CAD build for the part. Positions are in the model's coordinates, mm. A direction names the side the tool comes from. Round coordinates to 2 decimals unless told otherwise and drop trailing zeros. Write each loop counter-clockwise with the first axis right and the second up, starting at its lowest first coordinate (ties: lowest second). Pieces come first, ordered by that corner, then holes. Notation, with made-up numbers: (76, 74) -> (119, 74) arc R28 ccw to (119, 104) -> close; hole circle Ø8 at (5.5, 12). An arc over 180 degrees is marked (long way). Put each result on its own line as item: value. Start each with the question number.
1. Flat gauge pins, fed straight in: P1, Ø0.9, axis at y = 3.175, z = -50.8, coming from the +X side; P2, Ø0.8, axis at y = 3, z = -51, coming from the -X side; P3, Ø2, axis at x = 9.5, z = -13, coming from the -Y side. Where does each tip first touch, or does it go through?
2. Saw through at B-B on z = 0. List the corners of the cut face in (x, y).
3. Saw through at A-A on x = 0. List the corners of the cut face in (y, z).
4. Saw through at C-C on x = -15. List the corners of the cut face in (y, z), and give its area (3 significant figures).
5. Drill centre lines: line 1 (Z direction, x = 0, y = 5); line 2 (Y direction, x = 0, z = -70.75); line 3 (Z direction, x = 0, y = 4). Where is each one in solid material? Low to high. Write a range as from..to.
6. 3-axis set-ups, long thin cutter, end or side, ignore diameter. For faces 4 (the flat face through (-14, 6.35, -18)), 5 (the cylindrical face through (-0.93, 4.63, -73.07)): which of +Z, -Z, +X, -X, +Y, -Y reach the whole face in a straight line?
7. Pull direction Y, two halves, no side cores. Call faces 1 (the flat face through (58.75, 3, 1)), 2 (the flat face through (-14, 0, -18)), 3 (the flat face through (0, 3, -69.85)): pulls with the +Y half, pulls with the -Y half, needs draft (parallel to the pull), parting line crosses it, or undercut.
from build123d import *

# Parameters (mm, degrees)
SKETCH1_W           = 117.5004
SKETCH1_H           = 152.4
SKETCH1_R           = 19.05
BOSS_EXTRUDE1_DEPTH = 6.35
SKETCH3_R           = 0.7874
CUT_EXTRUDE1_DEPTH  = 0.508
SKETCH4_R           = 0.7874
CUT_EXTRUDE2_DEPTH  = 0.508
SKETCH5_R           = 1.7272
CUT_EXTRUDE3_DEPTH  = 6.35


with BuildPart() as part:
    # Sketch1 → Boss-Extrude1 (new body)
    with BuildSketch(Plane(origin=(0, 0, 0), x_dir=(1, 0, 0), z_dir=(0, 1, 0))):
        Rectangle(SKETCH1_W, SKETCH1_H)
        Circle(SKETCH1_R, mode=Mode.SUBTRACT)
    extrude(amount=BOSS_EXTRUDE1_DEPTH)

    # Sketch3 → Cut-Extrude1 (cut)
    with BuildSketch(Plane.ZY.offset(58.7502)):
        with Locations((-50.8, 3.175)):
            Circle(SKETCH3_R)
    extrude(amount=-CUT_EXTRUDE1_DEPTH, mode=Mode.SUBTRACT)

    # Sketch4 → Cut-Extrude2 (cut)
    with BuildSketch(Plane(origin=(58.7502, 0, 0), x_dir=(0, 0, -1), z_dir=(1, 0, 0))):
        with Locations((50.8, 3.175)):
            Circle(SKETCH4_R)
    extrude(amount=-CUT_EXTRUDE2_DEPTH, mode=Mode.SUBTRACT)

    # Sketch5 → Cut-Extrude3 (cut)
    with BuildSketch(Plane(origin=(0, 0, -76.2), x_dir=(-1, 0, 0), z_dir=(0, 0, -1))):
        with Locations((0, 3.175)):
            Circle(SKETCH5_R)
    extrude(amount=-CUT_EXTRUDE3_DEPTH, mode=Mode.SUBTRACT)


solid = part.part
Return value:
1. P1: stops at x = 58.24
1. P2: stops at x = -58.24
1. P3: passes through
2. outline: (-58.75, 0) -> (-19.05, 0) -> (-19.05, 6.35) -> (-58.75, 6.35) -> close; (19.05, 0) -> (58.75, 0) -> (58.75, 6.35) -> (19.05, 6.35) -> close
3. outline: (0, -76.2) -> (1.45, -76.2) -> (1.45, -69.85) -> (4.9, -69.85) -> (4.9, -76.2) -> (6.35, -76.2) -> (6.35, -19.05) -> (0, -19.05) -> close; (0, 19.05) -> (6.35, 19.05) -> (6.35, 76.2) -> (0, 76.2) -> close
4. outline: (0, -76.2) -> (6.35, -76.2) -> (6.35, -11.74) -> (0, -11.74) -> close; (0, 11.74) -> (6.35, 11.74) -> (6.35, 76.2) -> (0, 76.2) -> close
4. area: 819 mm^2
5. line 1: z = -76.2..-19.05, 19.05..76.2
5. line 2: y = 0..1.45, 4.9..6.35
5. line 3: z = -69.85..-19.05, 19.05..76.2
6. face 4: +Z, -Z, +X, -X, +Y
6. face 5: -Z
7. face 1: needs draft
7. face 2: pulls with the -Y half
7. face 3: undercut
